```python
from build123d import *

# Parameters (mm, degrees)
SKETCH1_W           = 11.8
SKETCH1_H           = 11.8
BOSS_EXTRUDE1_DEPTH = 11.8
SKETCH2_R           = 4.25
BOSS_EXTRUDE2_DEPTH = 1.5
SKETCH3_R           = 3.05
CUT_EXTRUDE1_DEPTH  = 9.5
SKETCH4_R           = 1.25
BOSS_EXTRUDE3_DEPTH = 8


with BuildPart() as part:
    # Sketch1 → Boss-Extrude1 (new body)
    with BuildSketch(Plane(origin=(0, 0, 0), x_dir=(1, 0, 0), z_dir=(0, 1, 0))):
        with Locations((5.9, 5.9)):
            Rectangle(SKETCH1_W, SKETCH1_H)
    extrude(amount=BOSS_EXTRUDE1_DEPTH)

    # Sketch2 → Boss-Extrude2 (add)
    with BuildSketch(Plane.XY):
        with Locations((5.9, 6.25)):
            Circle(SKETCH2_R)
    extrude(amount=BOSS_EXTRUDE2_DEPTH)

    # Sketch3 → Cut-Extrude1 (cut)
    with BuildSketch(Plane.XY.offset(1.5)):
        with Locations((5.9, 6.25)):
            Circle(SKETCH3_R)
    extrude(amount=-CUT_EXTRUDE1_DEPTH, mode=Mode.SUBTRACT)

    # Sketch4 → Boss-Extrude3 (add)
    with BuildSketch(Plane.XY.offset(-8)):
        with Locations((5.9, 6.25)):
            Circle(SKETCH4_R)
    extrude(amount=BOSS_EXTRUDE3_DEPTH)


solid = part.part
```
CAD build for the part. Positions are in the model's coordinates, mm. A direction names the side the tool comes from. Give positions to 0.01 mm unless a question says otherwise; leave off trailing zeros. Write each loop counter-clockwise with the first axis right and the second up, starting at its lowest first coordinate (ties: lowest second). Pieces come first, ordered by that corner, then holes. Notation, with made-up numbers: M 77,78.5 L 92,78.5 A9 cw 92,90.5 Z; hole C -1.5,-7.5 d9. An arc over 180 degrees is marked long. Return JSON: item names as keys, results as strings. Group by question number.
(1) Band-saw the part on A-A (z = -7). Give the cut face in (x, y), and give its area (3 significant figures).
(2) Flat gauge pins, fed straight in: pin 1 Ø5 at (x, z) = (7.5, -3) entering from -Y; pin 2 Ø0.8 at (x, y) = (6, 6) entering from +Z. Where does each tip first touch, or does it go through?
(3) Band-saw the part on D-D (z = 0.5). Give the cut face in (x, y), and give its area (3 significant figures).
(4) Band-saw the part on B-B (x = 5.9). Give the cut face in (y, z).
(5) Drill centre lines: L1, parallel to Y at x = 5.9, z = -4.75; L2, parallel to Y at x = 6.5, z = -5; L3, parallel to X at y = 6.5, z = -0.5. Where is each one in solid material? Low to high. Write a range as [from, to].
(6) 3-axis set-ups, long thin cutter, end or side, ignore diameter. For faces 1 (the face through (0, 6, -6)), 2 (the face through (6, 6, 0)): which of +Z, -Z, +X, -X, +Y, -Y reach the whole face in a straight line?
(7) Band-saw the part on C-C (y = 6.25). Give the cut face in (x, z).
(8) Mould opens along Y. For faces 3 (the face through (6, 11.8, -6)), 4 (the face through (5.239, 3.273, -3.183)), 5 (the face through (8, 3, 1.5)), 6 (the face through (7.2, 5.6, -8)) say: pulls with the +Y half, pulls with the -Y half, needs draft (parallel to the pull), parting line crosses it, or undercut.
Entries:
{
 "1": {"outline": "M 0,0 L 11.8,0 L 11.8,11.8 L 0,11.8 Z; C 5.9,6.25 d2.5; hole C 5.9,6.25 d6.1", "area": "115 mm^2"},
 "2": {"pin 1": "stops at y = 0", "pin 2": "stops at z = 0"},
 "3": {"outline": "C 5.9,6.25 d8.5; hole C 5.9,6.25 d6.1", "area": "27.5 mm^2"},
 "4": {"outline": "M 0,-11.8 L 11.8,-11.8 L 11.8,0 L 10.5,0 L 10.5,1.5 L 9.3,1.5 L 9.3,-8 L 7.5,-8 L 7.5,0 L 5,0 L 5,-8 L 3.2,-8 L 3.2,1.5 L 2,1.5 L 2,0 L 0,0 Z"},
 "5": {"L1": "y = [0, 3.2], [5, 7.5], [9.3, 11.8]", "L2": "y = [0, 3.26], [5.15, 7.35], [9.24, 11.8]", "L3": "x = [0, 2.86], [4.68, 7.12], [8.94, 11.8]"},
 "6": {"face 1": "+Z, -Z, -X, +Y, -Y", "face 2": "+Z"},
 "7": {"outline": "M 0,-11.8 L 11.8,-11.8 L 11.8,0 L 10.15,0 L 10.15,1.5 L 8.95,1.5 L 8.95,-8 L 7.15,-8 L 7.15,0 L 4.65,0 L 4.65,-8 L 2.85,-8 L 2.85,1.5 L 1.65,1.5 L 1.65,0 L 0,0 Z"},
 "8": {"face 3": "pulls with the +Y half", "face 4": "undercut", "face 5": "needs draft", "face 6": "undercut"}
}
